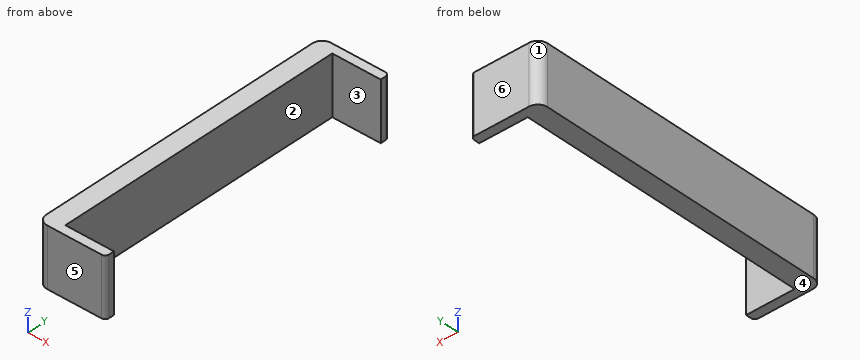
```python
from build123d import *

# Parameters (mm, degrees)
BOSS_EXTRUDE1_DEPTH = 30


with BuildPart() as part:
    # Sketch1 → Boss-Extrude1 (new body)
    with BuildSketch(Plane.XY):
        with BuildLine():
            Line((-17.5, 74.999850335), (-17.5, -74.999850335))
            ThreePointArc((-17.5, -74.999850335), (-16.035533906, -78.535384241), (-12.5, -79.999850335))
            Line((-12.5, -79.999850335), (15.5, -79.999850335))
            ThreePointArc((15.5, -79.999850335), (16.914213562, -79.414063897), (17.5, -77.999850335))
            Line((17.5, -77.999850335), (17.5, -75.249850335))
            Line((17.5, -75.249850335), (-7.5, -75.249850335))
            Line((-7.5, -75.249850335), (-7.5, 75.250149665))
            Line((-7.5, 75.250149665), (17.5, 75.250149665))
            Line((17.5, 75.250149665), (17.5, 77.999850335))
            ThreePointArc((17.5, 77.999850335), (16.914213562, 79.414063897), (15.5, 79.999850335))
            Line((15.5, 79.999850335), (-12.5, 79.999850335))
            ThreePointArc((-12.5, 79.999850335), (-16.035533906, 78.535384241), (-17.5, 74.999850335))
        make_face()
    extrude(amount=BOSS_EXTRUDE1_DEPTH)


solid = part.part
```
Verification items for the finished model (mm, model axes). Face numbers are marked on the shaded views. A direction names the side the tool comes from. Give positions to 0.01 mm unless a question says otherwise; leave off trailing zeros. Order: outer loops, then holes, each group sorted by start corner. A loop starts at its lowest first (then second) coordinate and runs counter-clockwise, first axis right, second up. Notation, with made-up numbers: M 69,3 L 116,3 A14 ccw 116,15 Z; hole C 48,-20.5 d9. An arc over 180 degrees is marked long. Return JSON: item names as keys, results as strings. Group by question number.
1) Section check B-B on z = 17.5. Record the cut outline in (x, y).
2) Access from +Z, -Z, +X, -X, +Y, -Y to the whole of each face (thin tool, end or side, straight path). Record for the marked faces 1 and 2.
3) Section check C-C on y = 23.5. Record the cut outline in (x, z).
4) Go/stop test with a flat-tipped pin: pin 1 Ø5 at (y, z) = (15.5, 13.5) entering from +X. Record where the tip stops, or that it passes through.
5) Mould release check, pull along Y, two halves, no side actions. Record for the marked faces 3, 4, 5 and 6: pulls with the +Y half, pulls with the -Y half, needs draft (parallel to the pull), parting line crosses it, or undercut.
6) Scan lines: line 1 (Y direction, x = 2.5, z = 18.75); line 2 (X direction, y = 28.5, z = 10.75); line 3 (Y direction, x = -13, z = 24.5). Record each from-to range of solid material in increasing order.
7) Section check A-A on x = 14. Record the cut outline in (y, z).
Answer block:
{
 "1": {"outline": "M -17.5,-75 A5 ccw -12.5,-80 L 15.5,-80 A2 ccw 17.5,-78 L 17.5,-75.25 L -7.5,-75.25 L -7.5,75.25 L 17.5,75.25 L 17.5,78 A2 ccw 15.5,80 L -12.5,80 A5 ccw -17.5,75 Z"},
 "2": {"face 1": "+Z, -Z, -X, +Y", "face 2": "+Z, -Z, +X"},
 "3": {"outline": "M -17.5,0 L -7.5,0 L -7.5,30 L -17.5,30 Z"},
 "4": {"pin 1": "stops at x = -7.5"},
 "5": {"face 3": "undercut", "face 4": "needs draft", "face 5": "pulls with the -Y half", "face 6": "pulls with the +Y half"},
 "6": {"line 1": "y = -80 to -75.25, 75.25 to 80", "line 2": "x = -17.5 to -7.5", "line 3": "y = -79.97 to 79.97"},
 "7": {"outline": "M -80,0 L -75.25,0 L -75.25,30 L -80,30 Z; M 75.25,0 L 80,0 L 80,30 L 75.25,30 Z"}
}
